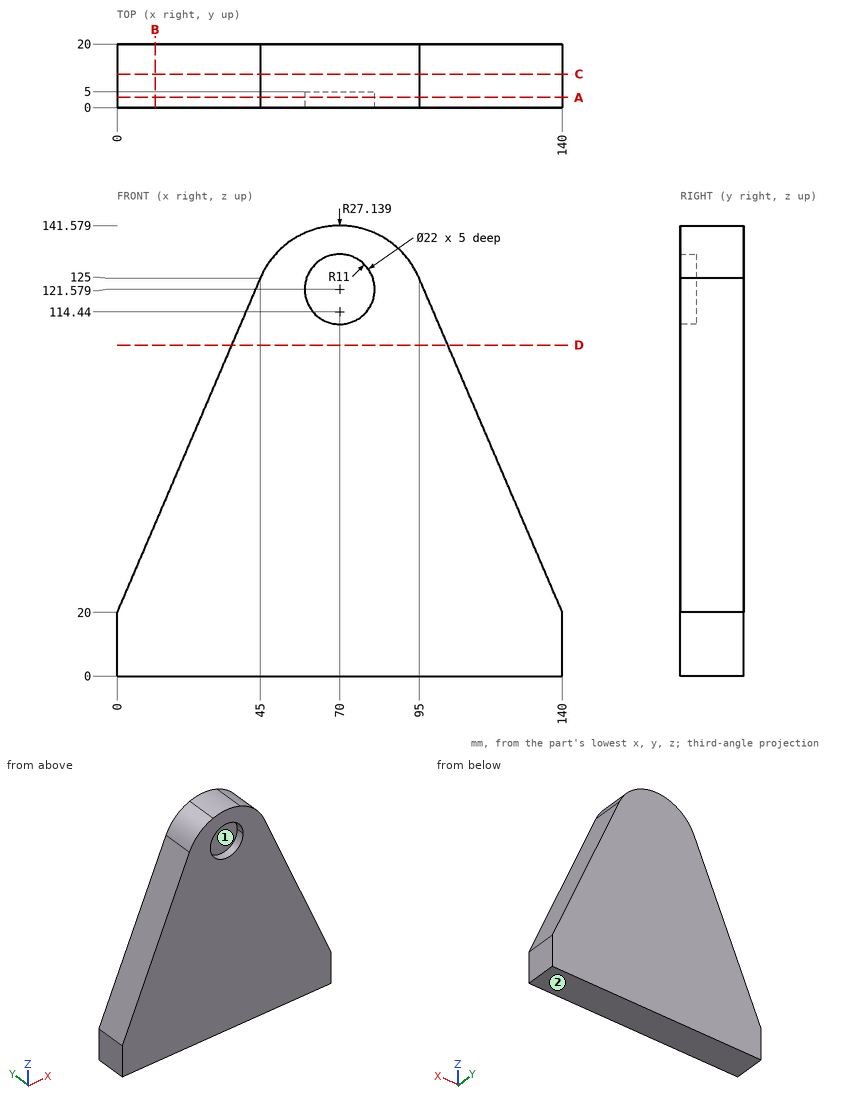
Geometry check sheet. Reference: drawing and pictorial views, mm from the part's lowest x, y, z. A direction names the side the tool comes from. Give positions to 0.01 mm unless a question says otherwise; leave off trailing zeros. Write each loop counter-clockwise with the first axis right and the second up, starting at its lowest first coordinate (ties: lowest second). Pieces come first, ordered by that corner, then holes. Notation, with made-up numbers: M 16.5,1.5 L 56.5,1.5 A24 ccw 56.5,18.5 Z; hole C 54.25,85.5 d10. An arc over 180 degrees is marked long. Answer as CSV lines item,"result". Start each with the question number.
Q1. Go/stop test with flat-tipped pins: pin 1 (3 mm diameter, centred on x = 35, y = 3, fed in from +Z) (1 decimal); pin 2 (1.5 mm diameter, centred on x = 83, y = 13, fed in from +Z); pin 3 (12 mm diameter, centred on y = 7, z = 29.5, fed in from +X). Record where each tip stops, or that it passes through.
Q2. Tool access check on the marked faces 1 and 2. Record the directions out of +Z, -Z, +X, -X, +Y, -Y that give a thin tool (end or side, any length) a straight path to the whole face; none if there is none.
Q3. Section check D-D, the plane z = 104. Record the cut outline in (x, y), then the cut area to 3 significant figures.
Q4. Material ranges on L1, parallel to Y at x = 80, z = 120; L2, parallel to X at y = 2, z = 61; L3, parallel to X at y = 5.5, z = 127.5, recorded low to high.
Q5. Section check A-A, the plane y = 3.25. Record the cut outline in (x, z), then the cut area to 3 significant figures.
Q6. Section check B-B, the plane x = 12. Record the cut outline in (y, z).
Q7. Section check C-C, the plane y = 10.5. Record the cut outline in (x, z), then the cut area to 3 significant figures.
Geometry says:
1,pin 1,"z = 105.2"
1,pin 2,"z = 138.66"
1,pin 3,"x = 138.5"
2,face 1,"-Y"
2,face 2,"-Z, +X, -X, +Y, -Y"
3,outline,"M 36,0 L 104,0 L 104,20 L 36,20 Z"
3,area,"1,360 mm^2"
4,L1,"5 to 20"
4,L2,"17.57 to 122.43"
4,L3,"46.21 to 93.79"
5,outline,"M 0,0 L 140,0 L 140,20 L 95,125 A27.14 ccw 45,125 L 0,20 Z; hole C 70,121.58 d22"
5,area,"13,000 mm^2"
6,outline,"M 0,0 L 20,0 L 20,48 L 0,48 Z"
7,outline,"M 0,0 L 140,0 L 140,20 L 95,125 A27.14 ccw 45,125 L 0,20 Z"
7,area,"13,400 mm^2"
